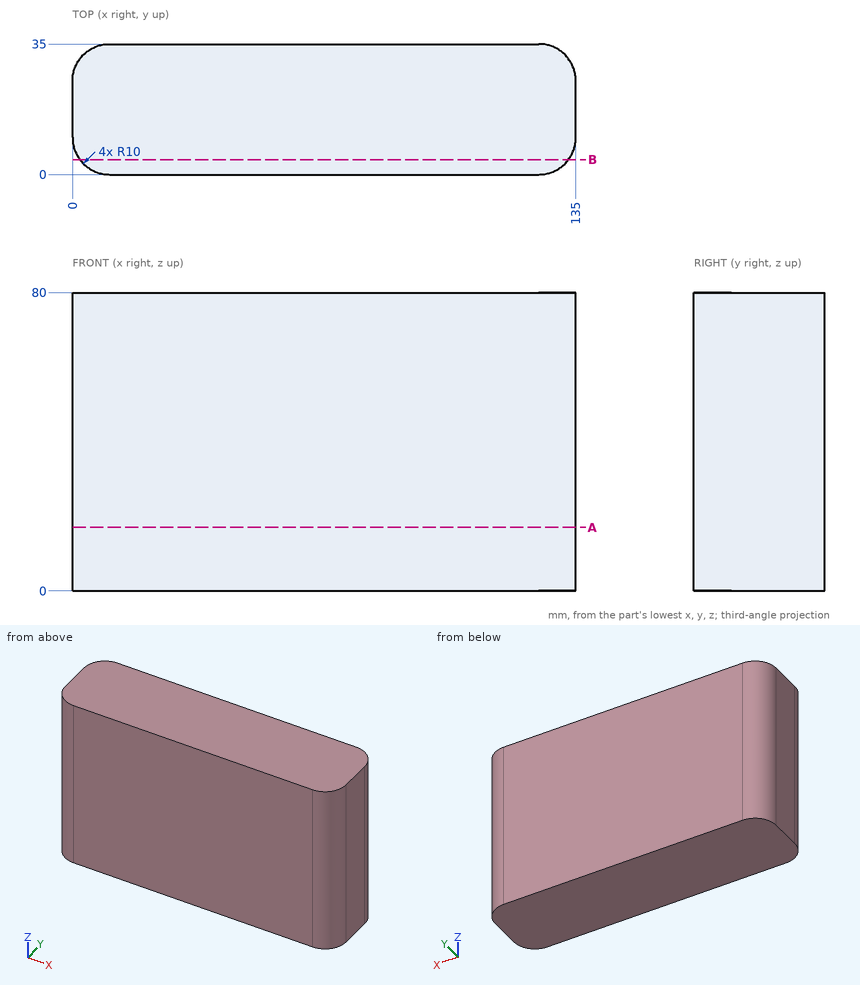
Verification items for this drawing (mm, ordinates from the low corner). Give positions to 0.01 mm unless a question says otherwise; leave off trailing zeros. Loops run counter-clockwise (first coordinate to the right, second up) from the corner with the lowest first, then second, coordinate; pieces in that order, holes last. Notation, with made-up numbers: M -29.5,9.25 L 9.5,9.25 A22 ccw 9.5,39.25 Z; hole C -29.5,1.25 d8. An arc over 180 degrees is marked long. Answer as CSV lines item,"result".
Item 1: Material ranges on line 1 (X direction, y = 25.5, z = 61.5); line 2 (X direction, y = 26.5, z = 57.5); line 3 (Y direction, x = 128.5, z = 67), recorded low to high.
Values:
line 1,"x = 0.01 to 134.99"
line 2,"x = 0.11 to 134.89"
line 3,"y = 0.63 to 34.37"
Item 2: Cross-section at A-A on z = 17. Record the cut outline in (x, y).
Values:
outline,"M 0,10 A10 ccw 10,0 L 125,0 A10 ccw 135,10 L 135,25 A10 ccw 125,35 L 10,35 A10 ccw 0,25 Z"
Item 3: Cross-section at B-B on y = 4. Record the cut outline in (x, z), and give its area (3 significant figures).
Values:
outline,"M 2,0 L 133,0 L 133,80 L 2,80 Z"
area,"10,500 mm²"
